Design review of the part built by this model. Coordinates are the model's own, in mm. A direction names the side the tool comes from. Give positions to 0.01 mm unless a question says otherwise; leave off trailing zeros. Loops run counter-clockwise (first coordinate to the right, second up) from the corner with the lowest first, then second, coordinate; pieces in that order, holes last. Notation, with made-up numbers: (-4, 50.25) -> (0, 50.25) arc R17 cw to (0, 58.25) -> close; hole circle Ø11 at (45.5, -13). An arc over 180 degrees is marked (long way). Answer as CSV lines item,"result".
Autodesk Inventor part; units mm, degrees
ref_plane "YZ Plane" through (0, 0, 0) normal (1, 0, 0) x (0, 1, 0)
ref_plane "XZ Plane" through (0, 0, 0) normal (0, 1, 0) x (-1, 0, 0)
ref_plane "XY Plane" through (0, 0, 0) normal (0, 0, 1) x (1, 0, 0)
sketch "Sketch1" plane through (0, 0, 0) normal (0, 0, 1) x (0, 1, 0)
  line L0 (98.3739, 70.6898) -> (232.7239, 70.6898)
  line L1 (238.7239, 64.6898) -> (238.7239, 56.6898)
  line L2 (244.7239, 50.6898) -> (352.7239, 50.6898)
  line L3 (358.7239, 56.6898) -> (358.7239, 64.6898)
  line L4 (364.7239, 70.6898) -> (499.0739, 70.6898)
  line L5 (505.0739, 64.6898) -> (505.0739, 21.6898)
  line L6 (499.0739, 15.6898) -> (470.0209, 15.6898)
  arc A0 (470.0209, 15.6898) -> (420.0521, -36.0749) centre (470.0209, -34.3102) ccw
  arc A1 (358.3704, -59.936) -> (420.0521, -36.0749) centre (385.0739, -37.3102) ccw
  arc A2 (358.3704, -59.936) -> (232.9093, -44.7528) centre (287.4489, -120.0273) ccw
  arc A3 (178.1588, -23.7808) -> (232.9093, -44.7528) centre (212.3739, -16.4102) ccw
  line L7 (129.28, 15.6898) -> (98.3739, 15.6898)
  line L8 (92.3739, 21.6898) -> (92.3739, 64.6898)
  circle A4 centre (212.3739, -16.4102) radius 17.5
  circle A5 centre (385.0739, -37.3102) radius 17.5
  arc A6 (178.1588, -23.7808) -> (129.28, 15.6898) centre (129.28, -34.3102) ccw
  arc A7 (92.3739, 21.6898) -> (98.3739, 15.6898) centre (98.3739, 21.6898) ccw
  arc A8 (98.3739, 70.6898) -> (92.3739, 64.6898) centre (98.3739, 64.6898) ccw
  arc A9 (238.7239, 64.6898) -> (232.7239, 70.6898) centre (232.7239, 64.6898) ccw
  arc A10 (238.7239, 56.6898) -> (244.7239, 50.6898) centre (244.7239, 56.6898) ccw
  arc A11 (352.7239, 50.6898) -> (358.7239, 56.6898) centre (352.7239, 56.6898) ccw
  arc A12 (364.7239, 70.6898) -> (358.7239, 64.6898) centre (364.7239, 64.6898) ccw
  arc A13 (505.0739, 64.6898) -> (499.0739, 70.6898) centre (499.0739, 64.6898) ccw
  arc A14 (499.0739, 15.6898) -> (505.0739, 21.6898) centre (499.0739, 21.6898) ccw
  point P0 (238.7239, 50.6898)
  point P1 (358.7239, 50.6898)
  point P2 (505.0739, 70.6898)
  point P3 (505.0739, 15.6898)
  dimension "d0" = 172.7
  dimension "d1" = 20.9
  dimension "d2" = 67.1
  dimension "d3" = 20
  dimension "d4" = 35
  dimension "d5" = 35
  dimension "d6" = 120
  dimension "d7" = 120
  dimension "d8" = 120
  dimension "d9" = 55
  dimension "d10" = 35
  dimension "d11" = 35
  dimension "d12" = 50
  dimension "d13" = 50
  dimension "d14" = 26.35
  dimension "d15" = 6
extrude "Extrusion1" add sketch "Sketch1" along normal blind 10
equation "\"d14\" = -0.5 * d6 + 0.5 * d0"
properties part number "3136 1133 83" material "Steel, Mild"
Q1. Clearance check with a flat-ended pin moving along its axis: pin 1 Ø6 at (x, z) = (-17, 1.5) entering from +Y. State where the tip first meets the part, or that it passes through.
Filled sheet:
pin 1,"stops at y = 504.83"
Q2. We need section B-B, the plane z = 8. State the section outline as (x, y) points.
Filled sheet:
outline,"(-70.69, 98.37) arc R6 ccw to (-64.69, 92.37) -> (-21.69, 92.37) arc R6 ccw to (-15.69, 98.37) -> (-15.69, 129.28) arc R50 cw to (23.78, 178.16) arc R35 ccw to (44.75, 232.91) arc R92.96 cw to (59.94, 358.37) arc R35 ccw to (36.07, 420.05) arc R50 cw to (-15.69, 470.02) -> (-15.69, 499.07) arc R6 ccw to (-21.69, 505.07) -> (-64.69, 505.07) arc R6 ccw to (-70.69, 499.07) -> (-70.69, 364.72) arc R6 ccw to (-64.69, 358.72) -> (-56.69, 358.72) arc R6 cw to (-50.69, 352.72) -> (-50.69, 244.72) arc R6 cw to (-56.69, 238.72) -> (-64.69, 238.72) arc R6 ccw to (-70.69, 232.72) -> close; hole circle Ø35 at (16.41, 212.37); hole circle Ø35 at (37.31, 385.07)"
Q3. We need section D-D, the plane x = 4.5. State the section outline as (y, z) points.
Filled sheet:
outline,"(169.42, 0) -> (199.55, 0) -> (199.55, 10) -> (169.42, 10) -> close; (225.2, 0) -> (429.88, 0) -> (429.88, 10) -> (225.2, 10) -> close"
Q4. To check wall thickness, follow probe 1 along Y at (x, z) = (34.5, 8.25); probe 2 along Y at (x, z) = (46, 3.75); probe 3 along Y at (x, z) = (-57, 1.25). State the ranges of each line that lie inside material, in increasing order. Write a range as from..to.
Filled sheet:
probe 1,"y = 182.41..251.04, 323.86..367.8, 402.35..420.02"
probe 2,"y = 193.68..231.07, 343.67..369.88, 400.26..418.98"
probe 3,"y = 92.37..238.72, 358.72..505.07"
Q5. We need section A-A, the plane y = 218.5. State the section outline as (x, z) points.
Filled sheet:
outline,"(-70.69, 0) -> (0.02, 0) -> (0.02, 10) -> (-70.69, 10) -> close; (32.8, 0) -> (50.87, 0) -> (50.87, 10) -> (32.8, 10) -> close"
Q6. We need section C-C, the plane x = 41. State the section outline as (y, z) points (3 decimals).
Filled sheet:
outline,"(187.467, 0) -> (238.505, 0) -> (238.505, 10) -> (187.467, 10) -> close; (336.393, 0) -> (367.967, 0) -> (367.967, 10) -> (336.393, 10) -> close; (402.18, 0) -> (419.879, 0) -> (419.879, 10) -> (402.18, 10) -> close"
Q7. For faces 4 (the flat face through (-50.69, 298, 5)), 5 (the flat face through (-15.69, 485, 5)), 6 (the cylindrical face through (27.633, 297.651, 4.93)), list the 3-axis set-ups (+Z, -Z, +X, -X, +Y, -Y) from which the entire face can be reached by the end or side of a thin tool; tool diameter is ignored.
Filled sheet:
face 4,"+Z, -Z, -X"
face 5,"+Z, -Z, +X, +Y"
face 6,"+Z, -Z, +X"
Q8. The part is to be moulded in two halves that separate along Y. For faces 1 (the flat face through (-43, 505.074, 5)), 2 (the cylindrical face through (21.785, 393.149, 4.93)), 3 (the flat face through (-15.69, 114, 5)), say which applies: pulls with the +Y half, pulls with the -Y half, needs draft (parallel to the pull), parting line crosses it, or undercut.
Filled sheet:
face 1,"pulls with the +Y half"
face 2,"undercut"
face 3,"needs draft"
